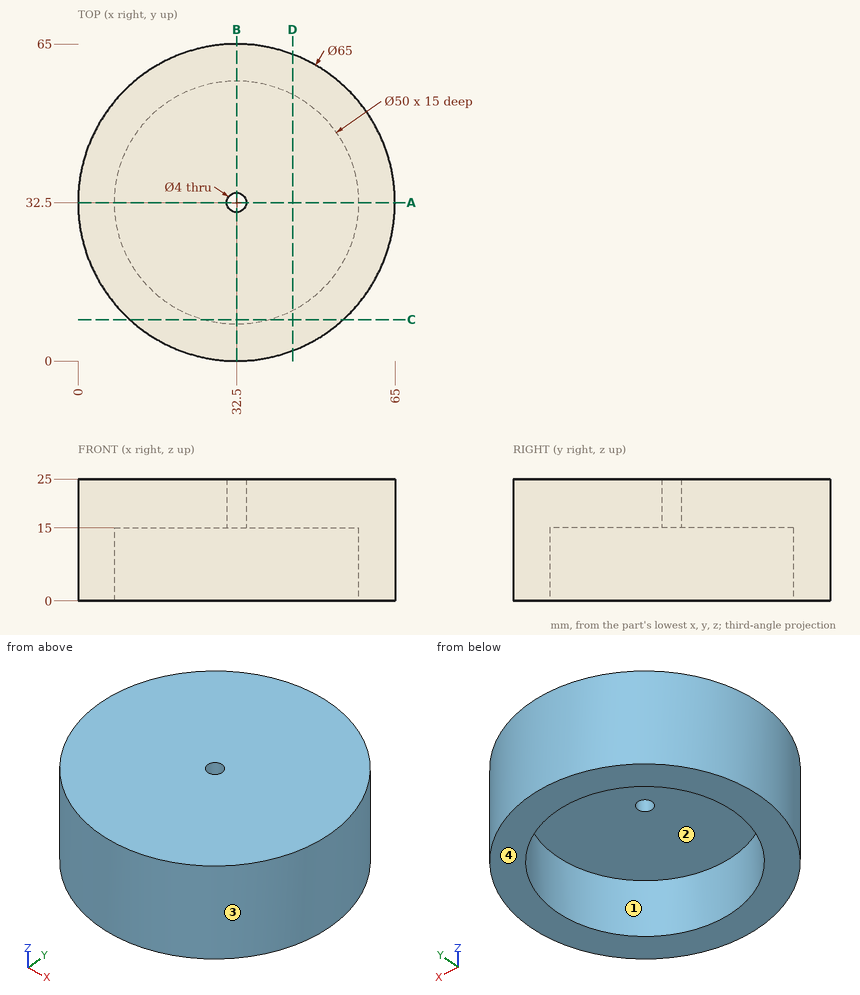
Verification items for this drawing (mm, ordinates from the low corner). Round coordinates to 2 decimals unless told otherwise and drop trailing zeros. Write each loop counter-clockwise with the first axis right and the second up, starting at its lowest first coordinate (ties: lowest second). Pieces come first, ordered by that corner, then holes. Notation, with made-up numbers: (81, 53) - (128, 53) arc R26 ccw to (128, 75) - close; hole circle Ø5 at (-14, 53.5). An arc over 180 degrees is marked (long way). Answer as a JSON object with one key per item and string values. Group by question number.
Q1. Section check A-A, the plane y = 32.5. Enter the section's corners in (x, z), plus the area to 3 significant figures.
Q2. Thickness scan on line 1 (Y direction, x = 32.5, z = 21.5); line 2 (Z direction, x = 45.5, y = 45); line 3 (X direction, y = 27.5, z = 7). Record the ranges inside material, lowest first.
Q3. Mould release check, pull along X, two halves, no side actions. Record for the marked faces 1, 2, 3 and 4: released by +X, released by -X, zero draft, split by the parting line, or undercut.
Q4. Section check D-D, the plane x = 44. Enter the section's corners in (y, z).
Q5. Section check C-C, the plane y = 8.5. Enter the section's corners in (x, z), plus the area to 3 significant figures.
Q6. Go/stop test with flat-tipped pins: pin 1 Ø8 at (x, z) = (22.5, 20) entering from -Y; pin 2 Ø15 at (x, y) = (36, 24.5) entering from -Z; pin 3 Ø2.5 at (x, y) = (32.5, 32.5) entering from -Z (1 decimal); pin 4 Ø6 at (x, z) = (10.5, 14) entering from +Y. Record where each tip stops, or that it passes through.
Found:
{
 "1": {"outline": "(0, 0) - (7.5, 0) - (7.5, 15) - (30.5, 15) - (30.5, 25) - (0, 25) - close; (34.5, 15) - (57.5, 15) - (57.5, 0) - (65, 0) - (65, 25) - (34.5, 25) - close", "area": "835 mm^2"},
 "2": {"line 1": "y = 0 to 30.5, 34.5 to 65", "line 2": "z = 15 to 25", "line 3": "x = 0.39 to 8.01, 56.99 to 64.61"},
 "3": {"face 1": "undercut", "face 2": "undercut", "face 3": "split by the parting line", "face 4": "zero draft"},
 "4": {"outline": "(2.1, 0) - (10.3, 0) - (10.3, 15) - (54.7, 15) - (54.7, 0) - (62.9, 0) - (62.9, 25) - (2.1, 25) - close"},
 "5": {"outline": "(10.59, 0) - (25.5, 0) - (25.5, 15) - (39.5, 15) - (39.5, 0) - (54.41, 0) - (54.41, 25) - (10.59, 25) - close", "area": "886 mm^2"},
 "6": {"pin 1": "stops at y = 0.56", "pin 2": "stops at z = 15", "pin 3": "passes through", "pin 4": "stops at y = 58.87"}
}
